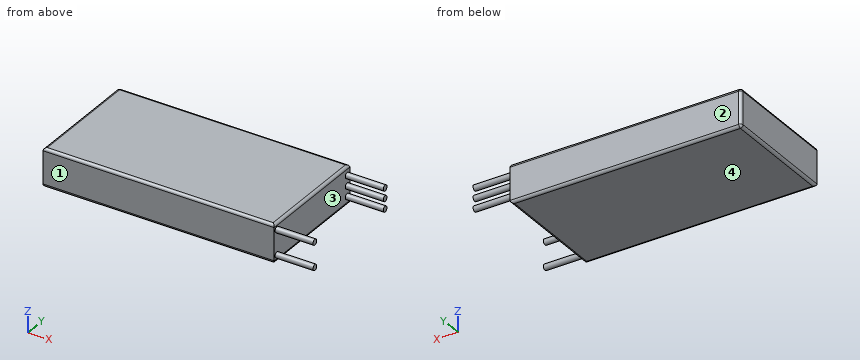
```python
from build123d import *

# Parameters (mm, degrees)
SKETCH1_W           = 71.12
SKETCH1_H           = 36.068
BOSS_EXTRUDE1_DEPTH = 11.684
SKETCH2_R           = 0.889
BOSS_EXTRUDE2_DEPTH = 11.684
FILLET1_R           = 0.8255


with BuildPart() as part:
    # Sketch1 → Boss-Extrude1 (new body)
    with BuildSketch(Plane.XY):
        with Locations((35.56, 18.034)):
            Rectangle(SKETCH1_W, SKETCH1_H)
    extrude(amount=BOSS_EXTRUDE1_DEPTH)

    # Sketch2 → Boss-Extrude2 (add)
    with BuildSketch(Plane(origin=(71.12, 0, 0), x_dir=(0, 0, -1), z_dir=(1, 0, 0))):
        with Locations(Location((-9.652, 1.27, 0), (0, 0, 180))):
            Circle(SKETCH2_R)
        with Locations(Location((-2.032, 1.27, 0), (0, 0, 180))):
            Circle(SKETCH2_R)
        with Locations(Location((-9.017, 34.798, 0), (0, 0, 180))):
            Circle(SKETCH2_R)
        with Locations(Location((-5.842, 34.798, 0), (0, 0, 180))):
            Circle(SKETCH2_R)
        with Locations(Location((-2.667, 34.798, 0), (0, 0, 180))):
            Circle(SKETCH2_R)
    extrude(amount=BOSS_EXTRUDE2_DEPTH)

    # Fillet1
    fillet1_edges = [part.edges().sort_by_distance(p)[0] for p in [
        (71.12, 18.034, 11.684),
        (35.56, 36.068, 11.684),
        (0, 18.034, 11.684),
        (35.56, 36.068, 0),
        (71.12, 18.034, 0),
        (35.56, 0, 0),
        (0, 18.034, 0),
        (0, 36.068, 5.842),
        (35.56, 0, 11.684),
    ]]
    fillet(fillet1_edges, radius=FILLET1_R)


solid = part.part
```
Input: part model. Units: mm. Frame: model coordinates. Face numbers are marked on the shaded views. Coordinates: 2 decimals unless noted, no trailing zeros. Order: outer loops, then holes, each group sorted by start corner. A loop starts at its lowest first (then second) coordinate and runs counter-clockwise, first axis right, second up. Notation, with made-up numbers: (-2, 59) - (53, 59) arc R28 cw to (53, 88) - close; hole circle Ø8 at (12, 65.25). An arc over 180 degrees is marked (long way). Put each result on its own line as item: value.
1. Line query: line 1 along X through (y, z) = (18.5, 9.25); line 2 along Y through (x, z) = (7.5, 0.75); line 3 along Z through (x, y) = (71, 30.5). Output: solid intervals per line, ascending.
Report:
line 1: x = 0 to 71.12
line 2: y = 0 to 36.06
line 3: z = 0.4 to 11.29
2. Cut plane A-A on y = 29. Return the cut outline in (x, z).
Report:
outline: (0, 0.83) arc R0.83 ccw to (0.83, 0) - (70.29, 0) arc R0.83 ccw to (71.12, 0.83) - (71.12, 10.86) arc R0.83 ccw to (70.29, 11.68) - (0.83, 11.68) arc R0.83 ccw to (0, 10.86) - close
3. Draft query along Y for the marked faces 1, 2, 3 and 4. Return one class per face: pulls with the +Y half, pulls with the -Y half, needs draft (parallel to the pull), parting line crosses it, or undercut.
Report:
face 1: pulls with the -Y half
face 2: pulls with the +Y half
face 3: undercut
face 4: needs draft
4. Contact query for a flat-ended pin moving along its axis: pin 1 Ø3 at (y, z) = (18.5, 4) entering from +X. Output: stop coordinate, or through.
Report:
pin 1: stops at x = 71.12
